For this review, take the finished solid that the model builds, in its own axes (mm). Coordinates: 2 decimals unless noted, no trailing zeros. Write each loop counter-clockwise with the first axis right and the second up, starting at its lowest first coordinate (ties: lowest second). Pieces come first, ordered by that corner, then holes. Notation, with made-up numbers: M 44,-31.5 L 60,-31.5 A9 cw 60,-14.5 Z; hole C 37,69 d11. An arc over 180 degrees is marked long. Return JSON: item names as keys, results as strings.
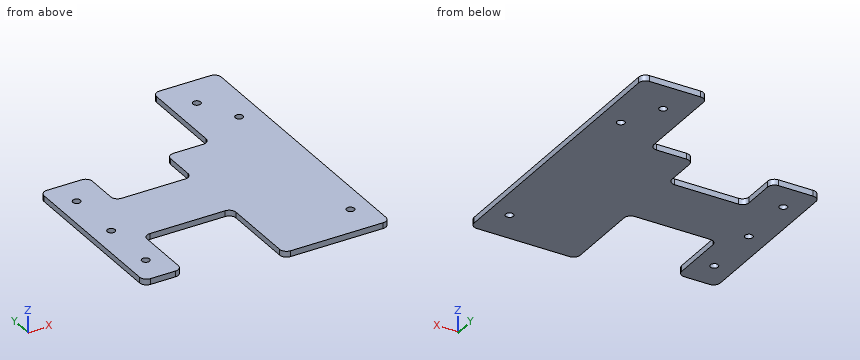
Autodesk Inventor part; units mm, degrees
ref_plane "YZ Plane" through (0, 0, 0) normal (1, 0, 0) x (0, 1, 0)
ref_plane "XZ Plane" through (0, 0, 0) normal (0, 1, 0) x (-1, 0, 0)
ref_plane "XY Plane" through (0, 0, 0) normal (0, 0, 1) x (1, 0, 0)
ref_plane "Work Plane1" through (678.6266, 4, 0) normal (0, 0, 1) x (1, 0, 0)
sketch "Sketch1" plane through (678.6266, 4, 0) normal (0, 0, 1) x (1, 0, 0)
  line L0 (0.5726, -1046.8384) -> (-66.4274, -1046.8384)
  line L1 (-109.4274, -1346.8384) -> (0.5726, -1346.8384)
  line L2 (0.5726, -1346.8384) -> (0.5726, -1046.8384)
  line L3 (-109.4274, -1256.8384) -> (-201.4274, -1256.8384)
  line L4 (-201.4274, -1256.8384) -> (-201.4274, -1324.8384)
  line L5 (-201.4274, -1324.8384) -> (-241.4274, -1324.8384)
  line L6 (-241.4274, -1324.8384) -> (-241.4274, -1144.8384)
  line L7 (-191.4274, -1190.8384) -> (-111.4274, -1190.8384)
  line L8 (-111.4274, -1146.8384) -> (-111.4274, -1190.8384)
  line L9 (-109.4274, -1256.8384) -> (-109.4274, -1346.8384)
  line L10 (-241.4274, -1144.8384) -> (-191.4274, -1144.8384)
  line L11 (-191.4274, -1144.8384) -> (-191.4274, -1190.8384)
  line L12 (-111.4274, -1146.8384) -> (-66.4274, -1146.8384)
  line L13 (-66.4274, -1146.8384) -> (-66.4274, -1046.8384)
  point P0 (-678.6266, -4)
  dimension "d0" = 110
  dimension "d4" = 92
  dimension "d5" = 68
  dimension "d6" = 40
  dimension "d7" = 180
  dimension "d8" = 50
  dimension "d9" = 46
  dimension "d10" = 300
  dimension "d12" = 80
  dimension "d13" = 44
  dimension "d14" = 45
  dimension "d15" = 100
extrude "Extrusion1" add sketch "Sketch1" along normal blind 6
fillet "Fillet1" radius 7 14 edges at (487.1992, -1186.8384, 3) (567.1992, -1186.8384, 3) (612.1992, -1042.8384, 3) (679.1992, -1042.8384, 3) (487.1992, -1140.8384, 3) (437.1992, -1140.8384, 3) (437.1992, -1320.8384, 3) (477.1992, -1320.8384, 3) (477.1992, -1252.8384, 3) (569.1992, -1252.8384, 3) (569.1992, -1342.8384, 3) (679.1992, -1342.8384, 3) (567.1992, -1142.8384, 3) (612.1992, -1142.8384, 3)
sketch "Sketch2" plane through (678.6266, 4, 6) normal (0, 0, 1) x (1, 0, 0)
  circle A0 centre (-221.4274, -1294.8384) radius 4
  circle A1 centre (-221.4274, -1234.8384) radius 4
  circle A2 centre (-221.4274, -1174.8384) radius 4
  line L0 (-234.4274, -1324.8384) -> (-208.4274, -1324.8384)
  line L1 (-221.4274, -1324.8384) -> (-221.4274, -1294.8384) construction
  line L2 (-221.4274, -1294.8384) -> (-221.4274, -1234.8384) construction
  line L3 (-221.4274, -1234.8384) -> (-221.4274, -1174.8384) construction
  line L4 (-241.4274, -1151.8384) -> (-241.4274, -1317.8384)
  line L5 (-241.4274, -1234.8384) -> (-221.4274, -1234.8384) construction
  circle A3 centre (-19.4274, -1311.8384) radius 4
  circle A4 centre (-21.4274, -1121.8384) radius 4
  circle A5 centre (-41.4274, -1081.8384) radius 4
  line L6 (-102.4274, -1346.8384) -> (-6.4274, -1346.8384)
  line L7 (0.5726, -1339.8384) -> (0.5726, -1053.8384)
  line L8 (-6.4274, -1046.8384) -> (-59.4274, -1046.8384)
  line L9 (-66.4274, -1053.8384) -> (-66.4274, -1139.8384)
  point P0 (-678.6266, -4)
  dimension "d17" = 8
  dimension "d18" = 60
  dimension "d19" = 60
  dimension "d20" = 8
  dimension "d21" = 35
  dimension "d22" = 20
  dimension "d23" = 35
  dimension "d24" = 25
  dimension "d25" = 40
  dimension "d26" = 20
  dimension "d27" = 30
extrude "Extrusion2" cut sketch "Sketch2" against normal through all
1. We need section B-B (z = 3.75). Give the number of separate pieces and of enclosed holes in the cut face, plus the area to 3 significant figures.
Checks:
{"separate pieces": "1", "enclosed holes": "6", "area": "42,200 mm2"}
2. We need section D-D (x = 500). State the section outline as (y, z) points, plus the area to 3 significant figures.
Checks:
{"outline": "M -1252.84,0 L -1186.84,0 L -1186.84,6 L -1252.84,6 Z", "area": "396 mm2"}
3. Clearance check with flat-ended pins moving along their axes: pin 1 Ø12 at (x, y) = (624.5, -1270.5) entering from -Z; pin 2 Ø1.8 at (y, z) = (-1104, 3) entering from -X; pin 3 Ø3 at (x, z) = (470.5, 2) entering from -Y; pin 4 Ø3 at (x, z) = (538, 3.5) entering from -Y. State where each tip first meets the part, or that it passes through.
Checks:
{"pin 1": "z = 0", "pin 2": "x = 612.2", "pin 3": "y = -1320.84", "pin 4": "y = -1252.84"}
4. Wall thickness on L1, parallel to X at y = -1282, z = 2.6; L2, parallel to X at y = -1294.5, z = 5.25; L3, parallel to X at y = -1311, z = 0.35: over which ranges is each line inside the solid? List them lowest first. Write a range as from..to.
Checks:
{"L1": "437.2..477.2, 569.2..679.2", "L2": "437.2..455.59, 458.81..477.2, 569.2..679.2", "L3": "437.2..477.2, 569.2..656.75, 661.65..679.2"}
5. We need section A-A (y = -1163). State the section outline as (x, z) points, plus the area to 3 significant figures.
Checks:
{"outline": "M 437.2,0 L 487.2,0 L 487.2,6 L 437.2,6 Z; M 567.2,0 L 679.2,0 L 679.2,6 L 567.2,6 Z", "area": "972 mm2"}
6. We need section C-C (y = -1263.5). State the section outline as (x, z) points.
Checks:
{"outline": "M 437.2,0 L 477.2,0 L 477.2,6 L 437.2,6 Z; M 569.2,0 L 679.2,0 L 679.2,6 L 569.2,6 Z"}
